Can you work these out from the model? Positions are in its coordinate system, mm. A direction names the side the tool comes from. Give positions to 0.01 mm unless a question says otherwise; leave off trailing zeros. Order: outer loops, then holes, each group sorted by start corner. A loop starts at its lowest first (then second) coordinate and runs counter-clockwise, first axis right, second up. Notation, with made-up numbers: (-0.75, 77) - (23.25, 77) arc R24 ccw to (23.25, 100) - close; hole circle Ø9 at (65.25, 69.25). An arc over 180 degrees is marked (long way). Return JSON: item names as keys, results as strings.
```python
from build123d import *

# Parameters (mm, degrees)
SKETCH1_R           = 4
BOSS_EXTRUDE1_DEPTH = 110
SKETCH2_R           = 7
BOSS_EXTRUDE2_DEPTH = 1
CHAMFER1_SIZE       = 3
FILLET1_R           = 8


with BuildPart() as part:
    # Sketch1 → Boss-Extrude1 (new body)
    with BuildSketch(Plane(origin=(0, 0, 0), x_dir=(1, 0, 0), z_dir=(0, 1, 0))):
        with Locations(Location((0, 0, 0), (0, 0, 270))):
            Circle(SKETCH1_R)
    extrude(amount=BOSS_EXTRUDE1_DEPTH)

    # Sketch2 → Boss-Extrude2 (add)
    with BuildSketch(Plane(origin=(0, 39, 0), x_dir=(-1, 0, 0), z_dir=(0, -1, 0))):
        with Locations(Location((0, 0, 0), (0, 0, 90))):
            Circle(SKETCH2_R)
    extrude(amount=-BOSS_EXTRUDE2_DEPTH)

    # Chamfer1
    chamfer1_edges = [part.edges().sort_by_distance(p)[0] for p in [
        (0, 39, -4),
    ]]
    chamfer(chamfer1_edges, length=CHAMFER1_SIZE - 0.0001)  # a hair under: the kernel refuses the full size

    # Fillet1
    fillet1_edges = [part.edges().sort_by_distance(p)[0] for p in [
        (0, 36.0001, -4),
    ]]
    fillet(fillet1_edges, radius=FILLET1_R)


solid = part.part
```
1. On a 3-axis mill with a long thin cutter (end or side, diameter ignored), from which of +Z, -Z, +X, -X, +Y, -Y can I reach the whole of each face in a straight line? I mean faces 1 (the face through (-3, 40, -3)), 2 (the face through (0, 0, 0)), 3 (the face through (-1.532, 16.114, 3.695)). Say none if no direction works.
Checks:
{"face 1": "+Y", "face 2": "+Z, -Z, +X, -X, -Y", "face 3": "-Y"}
2. Suppose I cut it at A-A (y = 11.5). List the corners of the cut face in (x, z) for me, plus the area to 3 significant figures.
Checks:
{"outline": "circle Ø8 at (0, 0)", "area": "50.3 mm^2"}
3. For pin 1 Ø4 at (x, z) = (0.5, 4) entering from -Y; pin 2 Ø1 at (y, z) = (89, 3.5) entering from -X; pin 3 Ø8 at (x, y) = (5, 94) entering from -Z; pin 4 Ø1 at (x, y) = (3.5, 31) entering from -Z, each with a flat end and sliding along its axis, tell me the tip position at first contact or that it passes through.
Checks:
{"pin 1": "y = 0", "pin 2": "x = -2.65", "pin 3": "z = -3.87", "pin 4": "z = -2.65"}
4. If I drill on L1, parallel to X at y = 30, z = -0.25; L2, parallel to Z at x = 0, y = 17.5; L3, parallel to Y at x = 0, z = -6, over which ranges is the centre line in solid material (lowest first)? Write a range as [from, to].
Checks:
{"L1": "[-3.99, 3.99]", "L2": "[-4, 4]", "L3": "[37.98, 40]"}
